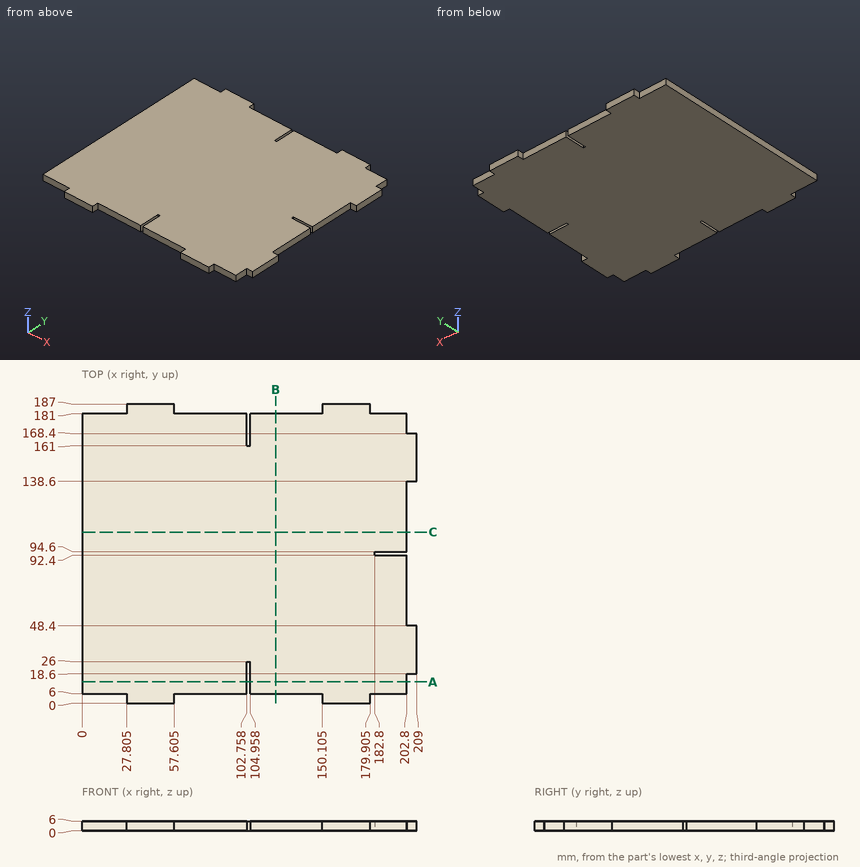
Could you check a few things on this drawing? It's one solid part, dimensions in mm from its lowest x, y, z. Give positions to 0.01 mm unless a question says otherwise; leave off trailing zeros. Order: outer loops, then holes, each group sorted by start corner. A loop starts at its lowest first (then second) coordinate and runs counter-clockwise, first axis right, second up. Notation, with made-up numbers: (66.5, 38) -> (89.5, 38) arc R20 cw to (89.5, 64) -> close; hole circle Ø4 at (23, 16). An arc over 180 degrees is marked (long way). Answer in a Markdown table with one row per item. Add a question column.
Item 1: Imagine slicing it at A-A (y = 13.5). List the corners of the cut face in (x, z) for me.
Item 2: Imagine slicing it at B-B (x = 121). List the corners of the cut face in (y, z) for me, and give its area (3 significant figures).
Item 3: Please list where these lines run through material, in increasing order: probe 1 along X at (y, z) = (23, 4.85); probe 2 along X at (y, z) = (179.5, 1.55); probe 3 along Y at (x, z) = (115.5, 5.75).
Item 4: I'm going to push flat-ended pins straight in: P1, Ø3, axis at x = 78, z = 3.5, coming from the +Y side; P2, Ø1.8, axis at y = 13, z = 4, coming from the +X side; P3, Ø0.7, axis at y = 94, z = 2, coming from the +X side. Where does each tip first touch, or does it pass through?
Item 5: Imagine slicing it at C-C (y = 107). List the corners of the cut face in (x, z) for me, and give its area (3 significant figures).
Result:
| question | item | result |
|---|---|---|
| 1 | outline | (0, 0) -> (102.76, 0) -> (102.76, 6) -> (0, 6) -> close; (104.96, 0) -> (202.8, 0) -> (202.8, 6) -> (104.96, 6) -> close |
| 2 | outline | (6, 0) -> (181, 0) -> (181, 6) -> (6, 6) -> close |
| 2 | area | 1,050 mm2 |
| 3 | probe 1 | 0 to 102.76, 104.96 to 209 |
| 3 | probe 2 | 0 to 102.76, 104.96 to 202.8 |
| 3 | probe 3 | 6 to 181 |
| 4 | P1 | y = 181 |
| 4 | P2 | x = 202.8 |
| 4 | P3 | x = 182.8 |
| 5 | outline | (0, 0) -> (202.8, 0) -> (202.8, 6) -> (0, 6) -> close |
| 5 | area | 1,220 mm2 |
